```python
from build123d import *

# Parameters (mm, degrees)
ESQUISSE1_R             = 17.5
BOSS_EXTRU_1_DEPTH      = 79.1
ESQUISSE2_R             = 6
BOSS_EXTRU_2_DEPTH      = 10
ESQUISSE3_R             = 3
BOSS_EXTRU_3_DEPTH      = 16.9
ESQUISSE4_W             = 6
ESQUISSE4_H             = 3
ENL_V_MAT_EXTRU_1_DEPTH = 5.5
D_GAGEMENT_M24_D        = 2.4
D_GAGEMENT_M24_DEPTH    = 10
D_GAGEMENT_M24_TIP      = 0.721032743


with BuildPart() as part:
    # Esquisse1 → Boss.-Extru.1 (new body)
    with BuildSketch(Plane.XY):
        Circle(ESQUISSE1_R)
    extrude(amount=BOSS_EXTRU_1_DEPTH)

    # Esquisse2 → Boss.-Extru.2 (add)
    with BuildSketch(Plane.XY.offset(79.1)):
        with Locations((0, 7)):
            Circle(ESQUISSE2_R)
    extrude(amount=BOSS_EXTRU_2_DEPTH)

    # Esquisse3 → Boss.-Extru.3 (add)
    with BuildSketch(Plane.XY.offset(89.1)):
        with Locations((0, 7)):
            Circle(ESQUISSE3_R)
    extrude(amount=BOSS_EXTRU_3_DEPTH)

    # Esquisse4 → Enlèv. mat.-Extru.1 (cut)
    with BuildSketch(Plane.XY.offset(106)):
        with Locations((0, 8.5)):
            Rectangle(ESQUISSE4_W, ESQUISSE4_H)
    extrude(amount=-ENL_V_MAT_EXTRU_1_DEPTH, mode=Mode.SUBTRACT)

    # Dégagement M24
    with Locations(Plane(origin=(13.40635523, 7.779436963, 79.1), x_dir=(1, 0, 0), z_dir=(0, 0, 1))):
        with Locations((0, 0), (-13.40635523, -23.279436963), (-26.829748989, -0.029436963)):
            Hole(D_GAGEMENT_M24_D / 2, depth=D_GAGEMENT_M24_DEPTH)
            with Locations((0, 0, -(D_GAGEMENT_M24_DEPTH + D_GAGEMENT_M24_TIP / 2))):  # 118° drill point
                Cone(0, D_GAGEMENT_M24_D / 2, D_GAGEMENT_M24_TIP, mode=Mode.SUBTRACT)


solid = part.part
```
Can you work these out from the model? Positions are in its coordinate system, mm. A direction names the side the tool comes from. Give positions to 0.01 mm unless a question says otherwise; leave off trailing zeros. Loops run counter-clockwise (first coordinate to the right, second up) from the corner with the lowest first, then second, coordinate; pieces in that order, holes last. Notation, with made-up numbers: M 70.5,-28 L 101.5,-28 A10 ccw 101.5,-10 Z; hole C 8,-15.5 d2. An arc over 180 degrees is marked long. Use one line per item in the form item = value. Start each with the question number.
(1) I'm going to push flat-ended pins straight in: P1, Ø3.5, axis at x = 0.5, y = 9, coming from the +Z side; P2, Ø1, axis at y = -10, z = 33, coming from the +X side; P3, Ø1, axis at x = -11.5, z = 70.5, coming from the +Y side. Where does each tip first touch, or does it pass through?
(2) On a 3-axis mill with a long thin cutter (end or side, diameter ignored), from which of +Z, -Z, +X, -X, +Y, -Y can I reach the whole of each face in a straight line? I mean faces 1 (the flat face through (1, 10, 89.1)), 2 (the flat face through (0, 8, 100.5)), 3 (the flat face through (0, 0, 0)). Say none if no direction works.
(3) I want a section at C-C, the plane x = 10. Write out the boundary of the cut face in (y, z), and give its area (3 significant figures).
(4) I want a section at A-A, the plane y = 11. Write out the boundary of the cut face in (x, z).
(5) Thinking about a two-plate mould opening in Y: for faces 4 (the flat face through (0, 0, 79.1)), 5 (the conical face through (-13.225, 7.813, 68.504)), 6 (the flat face through (0, 7, 103)), which applies, released by +Y, released by -Y, zero draft, split by the parting line, or undercut?
(6) I want a section at B-B, the plane z = 91. Write out the boundary of the cut face in (x, y).
(7) Please list where these lines run through material, in increasing order: line 1 (Y direction, x = 0, z = 72); line 2 (Z direction, x = 11, y = 13); line 3 (Z direction, x = -2.5, y = 12).
(8) I want a section at D-D, the plane y = 0. Write out the boundary of the cut face in (x, z).
Worked out:
q1.P1 = 100.5
q1.P2 = 14.7
q1.P3 = 13.61
q2.face_1 = +Z
q2.face_2 = +Z, +X, -X, +Y
q2.face_3 = -Z, +X, -X, +Y, -Y
q3.outline = M -14.36,0 L 14.36,0 L 14.36,79.1 L -14.36,79.1 Z
q3.area = 2,270 mm²
q4.outline = M -13.61,0 L 13.61,0 L 13.61,79.1 L 4.47,79.1 L 4.47,89.1 L -4.47,89.1 L -4.47,79.1 L -13.61,79.1 Z
q5.face_4 = zero draft
q5.face_5 = undercut
q5.face_6 = released by +Y
q6.outline = C 0,7 d6
q7.line_1 = -17.5 to -16.7, -14.3 to 17.5
q7.line_2 = 0 to 79.1
q7.line_3 = 0 to 89.1
q8.outline = M -17.5,0 L 17.5,0 L 17.5,79.1 L -17.5,79.1 Z
